Model file for the job. Use its own axes, mm. A direction names the side the tool comes from. Give positions to 0.01 mm unless a question says otherwise; leave off trailing zeros. Write each loop counter-clockwise with the first axis right and the second up, starting at its lowest first coordinate (ties: lowest second). Pieces come first, ordered by that corner, then holes.
```python
from build123d import *

# Parameters (mm, degrees)
PAD_DEPTH    = 3.5
POCKET_DEPTH = 8
FILLET_R     = 1


with BuildPart() as part:
    # Sketch → Pad (new body, symmetric)
    with BuildSketch(Plane.XZ):
        with BuildLine():
            Line((-40, 0), (0, 0))
            Line((0, 0), (0, 6))
            Line((0, 6), (-10, 6))
            Line((-10, 6), (-10, 2.8))
            ThreePointArc((-12, 0.8), (-10.585786, 1.385786), (-10, 2.8))
            Line((-12, 0.8), (-38, 0.8))
            ThreePointArc((-38, 0.8), (-39, 1.8), (-40, 0.8))
            Line((-40, 0.8), (-40, 0))
        make_face()
    extrude(amount=PAD_DEPTH, both=True)

    # Sketch001 → Pocket (cut)
    with BuildSketch(Plane(origin=(-10, 0, 0), x_dir=(0, 0, -1), z_dir=(-1, 0, 0))):
        Polygon((-6, -2.298131), (-6, 2.298131), (-5.224636, 2.298131), (-5.201471, 2.934012), (-2.171837, 2.934012), (-2.171837, -2.934012), (-5.224636, -2.934012), (-5.224636, -2.298131), align=None)
    extrude(amount=-POCKET_DEPTH, mode=Mode.SUBTRACT)

    # Fillet
    fillet_edges = [part.edges().sort_by_distance(p)[0] for p in [
        (0, -3.5, 3),
        (0, 3.5, 3),
    ]]
    fillet(fillet_edges, radius=FILLET_R)


solid = part.part
```
1. Pull direction Y, two halves, no side cores. Call faces 5 (the flat face through (-6, 0, 2.172)), 6 (the flat face through (-11.9, -3.5, 0.6)), 7 (the flat face through (-10, 3.2, 4.8)), 8 (the cylindrical face through (-0.301, 3.215, 3.042)): +Y half, -Y half, draft (parallel to the pull), parting line (faces both ways), or undercut.
Calculated:
face 5: undercut
face 6: -Y half
face 7: draft
face 8: +Y half
2. Slice it at B-B, the plane y = 1.5. Write the cut outline in (x, z).
Calculated:
outline: (-40, 0) - (0, 0) - (0, 6) - (-2, 6) - (-2, 2.17) - (-10, 2.17) - (-10, 2.8) arc R2 cw to (-12, 0.8) - (-38, 0.8) arc R1 ccw to (-40, 0.8) - close
3. Pin check, flat tips, straight feed: P1, Ø1, axis at y = 2.5, z = 4, coming from the -X side; P2, Ø3, axis at y = 1, z = 3.5, coming from the -X side. Stop position of each tip, or through.
Calculated:
P1: stops at x = -10
P2: stops at x = -10.17
4. Which spindle directions (+Z, -Z, +X, -X, +Y, -Y) get a long thin tool onto all of the face, cutting with end or side? Do faces 1 (the flat face through (0, 0, 3)), 2 (the flat face through (-6, -2.934, 4)), 3 (the flat face through (-10, -3.2, 4.8)), 4 (the flat face through (-25, 0, 0.8)). Say none if no direction does.
Calculated:
face 1: +Z, -Z, +X, +Y, -Y
face 2: none
face 3: +Z, -X, +Y, -Y
face 4: +Z, +Y, -Y
5. Slice it at C-C, the plane z = 3.9. Write the cut outline in (x, y).
Calculated:
outline: (-10, -3.5) - (-1, -3.5) arc R1 ccw to (0, -2.5) - (0, 2.5) arc R1 ccw to (-1, 3.5) - (-10, 3.5) - (-10, 2.93) - (-2, 2.93) - (-2, -2.93) - (-10, -2.93) - close
6. Slice it at A-A, the plane z = 1.3. Write the cut outline in (x, y), and give its area (3 significant figures).
Calculated:
outline: (-39.87, -3.5) - (-38.13, -3.5) - (-38.13, 3.5) - (-39.87, 3.5) - close; (-10.68, -3.5) - (-1, -3.5) arc R1 ccw to (0, -2.5) - (0, 2.5) arc R1 ccw to (-1, 3.5) - (-10.68, 3.5) - close
area: 86.4 mm2
7. Probe probe 1 along Z at (x, y) = (-3, 2.5); probe 2 along Y at (x, z) = (-6, 5.65); probe 3 along Y at (x, z) = (-2.5, 3.05). List the from-to ranges inside material, lowest first.
Calculated:
probe 1: z = 0 to 2.17, 5.22 to 6
probe 2: y = -3.5 to -2.3, 2.3 to 3.5
probe 3: y = -3.5 to -2.93, 2.93 to 3.5
8. Slice it at D-D, the plane x = -15.5. Write the cut outline in (y, z).
Calculated:
outline: (-3.5, 0) - (3.5, 0) - (3.5, 0.8) - (-3.5, 0.8) - close
